from build123d import *

# Parameters (mm, degrees)
SKETCH2_W           = 100
SKETCH2_H           = 120
BOSS_EXTRUDE1_DEPTH = 5
SKETCH3_W           = 5
SKETCH3_H           = 120
BOSS_EXTRUDE2_DEPTH = 125
SKETCH4_W           = 90
SKETCH4_H           = 5
BOSS_EXTRUDE3_DEPTH = 125
SKETCH5_W           = 10
SKETCH5_H           = 10
BOSS_EXTRUDE4_DEPTH = 15
SKETCH6_R           = 1.45
CUT_EXTRUDE1_DEPTH  = 10
CHAMFER1_SIZE       = 10
CUT_EXTRUDE2_DEPTH  = 10
SKETCH8_W           = 25
SKETCH8_H           = 65
CUT_EXTRUDE3_DEPTH  = 10
SKETCH9_R           = 1.75
CUT_EXTRUDE4_DEPTH  = 10
CUT_EXTRUDE5_DEPTH  = 10
BOSS_EXTRUDE5_START = 20
BOSS_EXTRUDE5_DEPTH = 20
SKETCH12_W          = 1
SKETCH12_H          = 6
CUT_EXTRUDE6_DEPTH  = 40
CHAMFER2_SIZE       = 1
SKETCH13_R          = 2.5
SKETCH13_R_2        = 1.45
BOSS_EXTRUDE6_DEPTH = 3
CHAMFER3_SIZE       = 3
SKETCH14_W          = 20
SKETCH14_H          = 25
CUT_EXTRUDE7_DEPTH  = 10
FILLET1_R           = 10


with BuildPart() as part:
    # Sketch2 → Boss-Extrude1 (new body)
    with BuildSketch(Plane(origin=(0, 0, 0), x_dir=(1, 0, 0), z_dir=(0, 1, 0))):
        with Locations((50, 60)):
            Rectangle(SKETCH2_W, SKETCH2_H)
    extrude(amount=BOSS_EXTRUDE1_DEPTH)

    # Sketch3 → Boss-Extrude2 (add)
    with BuildSketch(Plane.XZ):
        with Locations((97.5, -60)):
            Rectangle(SKETCH3_W, SKETCH3_H)
    extrude(amount=BOSS_EXTRUDE2_DEPTH)

    # Sketch4 → Boss-Extrude3 (add)
    with BuildSketch(Plane.XZ):
        with Locations((50, -2.5)):
            Rectangle(SKETCH4_W, SKETCH4_H)
    extrude(amount=BOSS_EXTRUDE3_DEPTH)

    # Sketch5 → Boss-Extrude4 (add)
    with BuildSketch(Plane.XZ.offset(125)):
        with Locations((90, -10)):
            Rectangle(SKETCH5_W, SKETCH5_H)
        with Locations((90, -110)):
            Rectangle(SKETCH5_W, SKETCH5_H)
    extrude(amount=-BOSS_EXTRUDE4_DEPTH)

    # Sketch6 → Cut-Extrude1 (cut)
    with BuildSketch(Plane.XZ.offset(125)):
        with Locations(Location((90, -10, 0), (0, 0, 270))):
            Circle(SKETCH6_R)
        with Locations(Location((90, -110, 0), (0, 0, 270))):
            Circle(SKETCH6_R)
    extrude(amount=-CUT_EXTRUDE1_DEPTH, mode=Mode.SUBTRACT)

    # Chamfer1
    chamfer1_edges = [part.edges().sort_by_distance(p)[0] for p in [
        (95, -110, -110),
        (95, -110, -10),
    ]]
    chamfer(chamfer1_edges, length=CHAMFER1_SIZE - 0.0001)  # a hair under: the kernel refuses the full size

    # Sketch7 → Cut-Extrude2 (cut)
    with BuildSketch(Plane.XZ):
        with BuildLine():
            Line((20, -7.5), (80, -7.5))
            ThreePointArc((80, -7.5), (82.5, -10), (80, -12.5))
            Line((80, -12.5), (20, -12.5))
            ThreePointArc((20, -12.5), (17.5, -10), (20, -7.5))
        make_face()
        with BuildLine():
            Line((20, -17.5), (80, -17.5))
            ThreePointArc((80, -17.5), (82.5, -20), (80, -22.5))
            Line((80, -22.5), (20, -22.5))
            ThreePointArc((20, -22.5), (17.5, -20), (20, -17.5))
        make_face()
        with BuildLine():
            Line((20, -27.5), (80, -27.5))
            ThreePointArc((80, -27.5), (82.5, -30), (80, -32.5))
            Line((80, -32.5), (20, -32.5))
            ThreePointArc((20, -32.5), (17.5, -30), (20, -27.5))
        make_face()
        with BuildLine():
            Line((20, -37.5), (80, -37.5))
            ThreePointArc((80, -37.5), (82.5, -40), (80, -42.5))
            Line((80, -42.5), (20, -42.5))
            ThreePointArc((20, -42.5), (17.5, -40), (20, -37.5))
        make_face()
        with BuildLine():
            Line((20, -47.5), (80, -47.5))
            ThreePointArc((80, -47.5), (82.5, -50), (80, -52.5))
            Line((80, -52.5), (20, -52.5))
            ThreePointArc((20, -52.5), (17.5, -50), (20, -47.5))
        make_face()
        with BuildLine():
            Line((20, -57.5), (80, -57.5))
            ThreePointArc((80, -57.5), (82.5, -60), (80, -62.5))
            Line((80, -62.5), (20, -62.5))
            ThreePointArc((20, -62.5), (17.5, -60), (20, -57.5))
        make_face()
        with BuildLine():
            Line((20, -67.5), (80, -67.5))
            ThreePointArc((80, -67.5), (82.5, -70), (80, -72.5))
            Line((80, -72.5), (20, -72.5))
            ThreePointArc((20, -72.5), (17.5, -70), (20, -67.5))
        make_face()
        with BuildLine():
            Line((20, -77.5), (80, -77.5))
            ThreePointArc((80, -77.5), (82.5, -80), (80, -82.5))
            Line((80, -82.5), (20, -82.5))
            ThreePointArc((20, -82.5), (17.5, -80), (20, -77.5))
        make_face()
        with BuildLine():
            Line((20, -87.5), (80, -87.5))
            ThreePointArc((80, -87.5), (82.5, -90), (80, -92.5))
            Line((80, -92.5), (20, -92.5))
            ThreePointArc((20, -92.5), (17.5, -90), (20, -87.5))
        make_face()
        with BuildLine():
            Line((20, -97.5), (80, -97.5))
            ThreePointArc((80, -97.5), (82.5, -100), (80, -102.5))
            Line((80, -102.5), (20, -102.5))
            ThreePointArc((20, -102.5), (17.5, -100), (20, -97.5))
        make_face()
        with BuildLine():
            Line((20, -107.5), (80, -107.5))
            ThreePointArc((80, -107.5), (82.5, -110), (80, -112.5))
            Line((80, -112.5), (20, -112.5))
            ThreePointArc((20, -112.5), (17.5, -110), (20, -107.5))
        make_face()
    extrude(amount=-CUT_EXTRUDE2_DEPTH, mode=Mode.SUBTRACT)

    # Sketch8 → Cut-Extrude3 (cut)
    with BuildSketch(Plane.XY):
        with Locations((17.5, -92.5)):
            Rectangle(SKETCH8_W, SKETCH8_H)
    extrude(amount=-CUT_EXTRUDE3_DEPTH, mode=Mode.SUBTRACT)

    # Sketch9 → Cut-Extrude4 (cut)
    with BuildSketch(Plane.XZ):
        with Locations(Location((10, -110, 0), (0, 0, 270))):
            Circle(SKETCH9_R)
        with Locations(Location((10, -10, 0), (0, 0, 270))):
            Circle(SKETCH9_R)
        with Locations(Location((90, -110, 0), (0, 0, 270))):
            Circle(SKETCH9_R)
    extrude(amount=-CUT_EXTRUDE4_DEPTH, mode=Mode.SUBTRACT)

    # Sketch10 → Cut-Extrude5 (cut)
    with BuildSketch(Plane.XZ):
        with BuildLine():
            Line((6, -95), (6, -80))
            ThreePointArc((6, -80), (11, -75), (16, -80))
            Line((16, -80), (16, -95))
            ThreePointArc((16, -95), (11, -100), (6, -95))
        make_face()
    extrude(amount=-CUT_EXTRUDE5_DEPTH, mode=Mode.SUBTRACT)

    # Sketch11 → Boss-Extrude5 (add)
    with BuildSketch(Plane.XZ.offset(BOSS_EXTRUDE5_START)):
        with BuildLine():
            ThreePointArc((6, -80), (11, -71.923580655), (16, -80))
            ThreePointArc((16, -80), (11, -75), (6, -80))
        make_face()
    extrude(amount=-BOSS_EXTRUDE5_DEPTH)

    # Sketch12 → Cut-Extrude6 (cut)
    with BuildSketch(Plane(origin=(0, 0, 0), x_dir=(0, 0, -1), z_dir=(1, 0, 0))):
        with Locations((72.423580655, -10)):
            Rectangle(SKETCH12_W, SKETCH12_H)
    extrude(amount=CUT_EXTRUDE6_DEPTH, mode=Mode.SUBTRACT)

    # Chamfer2
    chamfer2_edges = [part.edges().sort_by_distance(p)[0] for p in [
        (11, -13, -72.923580655),
        (11, -7, -72.923580655),
    ]]
    chamfer(chamfer2_edges, length=CHAMFER2_SIZE - 0.0001)  # a hair under: the kernel refuses the full size

    # Sketch13 → Boss-Extrude6 (add)
    # profile 1 of 4: a face of its own
    with BuildSketch(Plane.ZY.offset(-95)):
        with Locations(Location((-97.9, -110.9, 0), (0, 0, 180))):
            Circle(SKETCH13_R)
        with Locations((-97.9, -110.9)):
            Circle(SKETCH13_R_2, mode=Mode.SUBTRACT)
    # profile 2 of 4: a face of its own
    with BuildSketch(Plane.ZY.offset(-95)):
        with Locations(Location((-97.9, -9.1, 0), (0, 0, 180))):
            Circle(SKETCH13_R)
        with Locations((-97.9, -9.1)):
            Circle(SKETCH13_R_2, mode=Mode.SUBTRACT)
    # profile 3 of 4: a face of its own
    with BuildSketch(Plane.ZY.offset(-95)):
        with Locations(Location((-22.1, -9.1, 0), (0, 0, 180))):
            Circle(SKETCH13_R)
        with Locations((-22.1, -9.1)):
            Circle(SKETCH13_R_2, mode=Mode.SUBTRACT)
    # profile 4 of 4: a face of its own
    with BuildSketch(Plane.ZY.offset(-95)):
        with Locations(Location((-22.1, -110.9, 0), (0, 0, 180))):
            Circle(SKETCH13_R)
        with Locations((-22.1, -110.9)):
            Circle(SKETCH13_R_2, mode=Mode.SUBTRACT)
    extrude(amount=BOSS_EXTRUDE6_DEPTH)

    # Chamfer3
    chamfer3_edges = [part.edges().sort_by_distance(p)[0] for p in [
        (95, -110.9, -95.4),
        (95, -9.1, -95.4),
        (95, -9.1, -19.6),
        (95, -110.9, -19.6),
    ]]
    chamfer(chamfer3_edges, length=CHAMFER3_SIZE - 0.0001)  # a hair under: the kernel refuses the full size

    # Sketch14 → Cut-Extrude7 (cut)
    with BuildSketch(Plane(origin=(0, 0, -5), x_dir=(-1, 0, 0), z_dir=(0, 0, -1))):
        with Locations((-85, -87.5)):
            Rectangle(SKETCH14_W, SKETCH14_H)
    extrude(amount=-CUT_EXTRUDE7_DEPTH, mode=Mode.SUBTRACT)

    # Fillet1
    fillet1_edges = [part.edges().sort_by_distance(p)[0] for p in [
        (30, -60, -2.5),
        (75, -75, -2.5),
        (75, -100, -2.5),
    ]]
    fillet(fillet1_edges, radius=FILLET1_R)


solid = part.part
Build history of the part. All positions in model axes, mm. A direction names the side the tool comes from. Give positions to 0.01 mm unless a question says otherwise; leave off trailing zeros. Loops run counter-clockwise (first coordinate to the right, second up) from the corner with the lowest first, then second, coordinate; pieces in that order, holes last. Notation, with made-up numbers: (67.25, -0.75) - (112.25, -0.75) arc R20 ccw to (112.25, 16.25) - close; hole circle Ø9 at (31, 43). An arc over 180 degrees is marked (long way). Write item = value, one per line. Start each with the question number.
1) Probe probe 1 along Z at (x, y) = (90, -121); probe 2 along Z at (x, y) = (93, -110); probe 3 along Y at (x, z) = (94.4, -22.1). List the from-to ranges inside material, lowest first. Write a range as from..to.
2) Band-saw the part on B-B on x = 34. Count the separate pieces of the cut face and the enclosed holes in it, plus the area to 3 significant figures.
3) Drop flat-ended pins along their axis: pin 1 Ø5 at (x, z) = (29, -54.5) entering from -Y; pin 2 Ø12 at (x, y) = (70.5, -32) entering from -Z; pin 3 Ø0.9 at (x, z) = (90, -9.5) entering from -Y. Give the stop position or say it passes through.
4) Band-saw the part on A-A on z = -40. Give the cut face in (x, y).
5) Band-saw the part on C-C on y = -28. Give the cut face in (x, z), plus the area to 3 significant figures.
6) Band-saw the part on D-D on y = -72.5. Give the cut face in (x, z), plus the area to 3 significant figures.
7) Pull direction X, two halves, no side cores. Call faces 1 (the flat face through (90, -115, -15)), 2 (the cylindrical face through (88.29, 2.46, -109.62)), 3 (the conical face through (92.146, -109.29, -95.8)): +X half, -X half, draft (parallel to the pull), parting line (faces both ways), or undercut.
8) Tool access for faces 4 (the flat face through (11, -20, -74)), 5 (the cylindrical face through (17.5, 2.5, -90.1)), 6 (the flat face through (11, -10, -72.924)): list every direction of +Z, -Z, +X, -X, +Y, -Y with a clear straight run to the whole face (end or side of a thin tool).
Final values:
q1.probe_1 = -115..-111.45, -108.55..-105, -15..-11.45, -8.55..0
q1.probe_2 = -115..-105, -101.28..-99.04, -96.76..-94.52, -25.48..-23.24, -20.96..-18.72, -15..0
q1.probe_3 = -115.8..-112.35, -109.45..-106, -14..-10.55, -7.65..-4.2, 0..5
q2.separate_pieces = 12
q2.enclosed_holes = 0
q2.area = 950 mm²
q3.pin_1 = 0
q3.pin_2 = -5
q3.pin_3 = -115
q4.outline = (0, 0) - (17.5, 0) - (17.5, 5) - (0, 5) - close; (82.5, 0) - (95, 0) - (95, -125) - (100, -125) - (100, 5) - (82.5, 5) - close
q5.outline = (5, -5) - (95, -5) - (95, -120) - (100, -120) - (100, 0) - (5, 0) - close
q5.area = 1,050 mm²
q6.outline = (30, -5) - (95, -5) - (95, -120) - (100, -120) - (100, 0) - (30, 0) - close
q6.area = 925 mm²
q7.face_1 = draft
q7.face_2 = undercut
q7.face_3 = -X half
q8.face_4 = -Z, -X, -Y
q8.face_5 = +Y, -Y
q8.face_6 = -X
